Source: CAD feature listing. Evaluate the final solid. Frame: model axes, mm. A direction names the side the tool comes from. Round coordinates to 2 decimals unless told otherwise and drop trailing zeros. Loops run counter-clockwise (first coordinate to the right, second up) from the corner with the lowest first, then second, coordinate; pieces in that order, holes last. Notation, with made-up numbers: M -15,78 L 33,78 A22 cw 33,103 Z; hole C 62,6.5 d1. An arc over 180 degrees is marked long. Write each question's results on one line, items separated by ' | '. Start each with the question number.
1. Section A-A on x = 0. Output: boundary loops of the cut face in (y, z) (3 decimals).
2. Draft query along X for faces 3 (the flat face through (50, 0, 0)), 4 (the cylindrical face through (27.9, 1.27, -0.09)), 5 (the flat face through (-1, -1, -3.5)), 6 (the flat face through (-50, 0, 0)). Return one class per face: released by +X, released by -X, zero draft, split by the parting line, or undercut.
3. Section B-B on y = -1.35. Output: boundary loops of the cut face in (x, z).
4. Contact query for flat-ended pins moving along their axis: pin 1 Ø1.4 at (x, z) = (45, 0) entering from -Y; pin 2 Ø2.5 at (x, z) = (0, 0) entering from +Y; pin 3 Ø1 at (x, y) = (20, 1) entering from +Z. Output: stop coordinate, or through.
5. Ray query, line 1 (Z direction, x = -15, y = -0.8); line 2 (Z direction, x = 30, y = 0.8); line 3 (Y direction, x = -6.5, z = 2.75). Return the intervals inside material, ascending.
6. Section C-C on x = 27. Output: boundary loops of the cut face in (y, z) (3 decimals).
7. Set-up query: faces 1 (the cylindrical face through (-28.89, -1.13, 0.46)), 2 (the flat face through (44, 0.1, 1)). Return all of +Z, -Z, +X, -X, +Y, -Y with unobstructed straight access to the full face (end or side cutting, diameter ignored); none if empty.
from build123d import *

# Parameters (mm, degrees)
SKETCH_1_W             = 100
SKETCH_1_H             = 4.8
EXTRUDE_1_DEPTH        = 3.5
SKETCH_3_R             = 2.1
CUT_EXTRUDE_1_DEPTH    = 2.3
SKETCH_4_R             = 1.2
CUT_EXTRUDE_2_DEPTH    = 2.5
CUT_EXTRUDE_START      = -101
CUT_EXTRUDE_4_DEPTH    = 102
PATTERN_LINEAR_1_COUNT = 6
PATTERN_LINEAR_1_PITCH = 15


with BuildPart() as part:
    # 草图1 → 凸台-拉伸1 (new body, symmetric)
    with BuildSketch(Plane.XY):
        Rectangle(SKETCH_1_W, SKETCH_1_H)
    extrude(amount=EXTRUDE_1_DEPTH, both=True)

    # 草图3 → 切除-拉伸1 (cut)
    with BuildSketch(Plane(origin=(0, 2.4, 0), x_dir=(1, 0, 0), z_dir=(0, 1, 0))):
        with Locations((-45, 0)):
            Circle(SKETCH_3_R)
    cut_extrude_1 = extrude(amount=-CUT_EXTRUDE_1_DEPTH, mode=Mode.SUBTRACT)

    # 草图4 → 切除-拉伸2 (cut)
    with BuildSketch(Plane(origin=(0, 0.1, 0), x_dir=(1, 0, 0), z_dir=(0, 1, 0))):
        with Locations((-45, 0)):
            Circle(SKETCH_4_R)
    cut_extrude_2 = extrude(amount=-CUT_EXTRUDE_2_DEPTH, mode=Mode.SUBTRACT)

    # 镜向1: 切除-拉伸1, 切除-拉伸2 across plane
    add(cut_extrude_1.mirror(Plane(origin=(0, 0, 0), x_dir=(0, 0, 1), z_dir=(1, 0, 0))), mode=Mode.SUBTRACT)
    add(cut_extrude_2.mirror(Plane(origin=(0, 0, 0), x_dir=(0, 0, 1), z_dir=(1, 0, 0))), mode=Mode.SUBTRACT)

    # 草图6 → 切除-拉伸4 (cut)
    with BuildSketch(Plane.ZY.offset(50).offset(CUT_EXTRUDE_START)):
        with BuildLine():
            Line((3.5, 29.375276139), (3.5, 2.4))
            Line((3.5, 2.4), (3.5, 2.223915661))
            ThreePointArc((3.5, 2.223915661), (3.476466019, 2.072323667), (3.408079469, 1.935001925))
            Line((3.408079469, 1.935001925), (2.604516262, 0.8))
            Line((2.604516262, 0.8), (3.408079469, -0.335001925))
            ThreePointArc((3.408079469, -0.335001925), (3.476466019, -0.472323667), (3.5, -0.623915661))
            Line((3.5, -0.623915661), (3.5, -27.5991918))
            Line((3.5, -27.5991918), (57.450552278, -27.5991918))
            Line((57.450552278, -27.5991918), (57.450552278, 29.375276139))
            Line((57.450552278, 29.375276139), (3.5, 29.375276139))
        make_face()
    cut_extrude_4 = extrude(amount=CUT_EXTRUDE_4_DEPTH, mode=Mode.SUBTRACT)

    # 镜向3: 切除-拉伸4 across plane
    add(cut_extrude_4.mirror(Plane.XY), mode=Mode.SUBTRACT)

    # 阵列(线性)1: 切除-拉伸1, 切除-拉伸2 ×6
    with Locations(*[(i * PATTERN_LINEAR_1_PITCH, 0, 0) for i in range(1, PATTERN_LINEAR_1_COUNT)]):
        add(cut_extrude_1, mode=Mode.SUBTRACT)
        add(cut_extrude_2, mode=Mode.SUBTRACT)


solid = part.part
Taken from the geometry:
1) outline: M -2.4,-3.5 L -0.624,-3.5 A0.5 ccw -0.335,-3.408 L 0.8,-2.605 L 1.935,-3.408 A0.5 ccw 2.224,-3.5 L 2.4,-3.5 L 2.4,-2.1 L 0.1,-2.1 L 0.1,-1.2 L -2.4,-1.2 Z; M -2.4,1.2 L 0.1,1.2 L 0.1,2.1 L 2.4,2.1 L 2.4,3.5 L 2.224,3.5 A0.5 ccw 1.935,3.408 L 0.8,2.605 L -0.335,3.408 A0.5 ccw -0.624,3.5 L -2.4,3.5 Z
2) face 3: released by +X | face 4: undercut | face 5: zero draft | face 6: released by -X
3) outline: M -50,-3.5 L 50,-3.5 L 50,3.5 L -50,3.5 Z; hole C -45,0 d2.4; hole C -30,0 d2.4; hole C -15,0 d2.4; hole C 0,0 d2.4; hole C 15,0 d2.4; hole C 30,0 d2.4; hole C 45,0 d2.4
4) pin 1: through | pin 2: y = 0.1 | pin 3: z = 3.1
5) line 1: -3.5 to -1.2, 1.2 to 3.5 | line 2: -2.6 to -2.1, 2.1 to 2.6 | line 3: -2.4 to 0.59, 1.01 to 2.4
6) outline: M -2.4,-3.5 L -0.624,-3.5 A0.5 ccw -0.335,-3.408 L 0.8,-2.605 L 1.935,-3.408 A0.5 ccw 2.224,-3.5 L 2.4,-3.5 L 2.4,3.5 L 2.224,3.5 A0.5 ccw 1.935,3.408 L 0.8,2.605 L -0.335,3.408 A0.5 ccw -0.624,3.5 L -2.4,3.5 Z
7) face 1: +Y, -Y | face 2: +Y
